CAD build for the part. Positions are in the model's coordinates, mm. A direction names the side the tool comes from. Give positions to 0.01 mm unless a question says otherwise; leave off trailing zeros. Write each loop counter-clockwise with the first axis right and the second up, starting at its lowest first coordinate (ties: lowest second). Pieces come first, ordered by that corner, then holes. Notation, with made-up numbers: M 35.25,-39.75 L 83.25,-39.75 A16 cw 83.25,-13.75 Z; hole C -6.5,9 d1. An arc over 180 degrees is marked long. One line per question, with ' | ' between items. Start each with the question number.
1. Flat gauge pins, fed straight in: pin 1 (0.8 mm diameter, centred on y = -23, z = 1, fed in from +X); pin 2 (17.5 mm diameter, centred on x = -0.5, z = -36.5, fed in from +Y); pin 3 (17.5 mm diameter, centred on y = -7, z = -18, fed in from -X). Where does each tip first touch, or does it go through?
2. Cut at A-A, the plane y = 0. Count the separate pieces of the cut face and the enclosed holes in it, then the cut area to 3 significant figures.
3. Cut at B-B, the plane x = -40. Write the cut outline in (y, z).
4. Cut at D-D, the plane x = -7.5. Write the cut outline in (y, z), then the cut area to 3 significant figures.
5. Which spindle directions (+Z, -Z, +X, -X, +Y, -Y) get a long thin tool onto all of the face, cutting with end or side? Do faces 1 (the face through (0, -17.5, -34)), 2 (the face through (0, 20, -37)), 3 (the face through (20, 0, -37)), 4 (the face through (-20, 0, -37)), 5 (the face through (0, -20, -37)). Say none if no direction does.
6. Cut at C-C, the plane z = -55.5. Write the cut outline in (x, y).
7. Pull direction X, two halves, no side cores. Call faces 6 (the face through (-58, -4, 2.5)), 7 (the face through (60, -1, 5)), 8 (the face through (-35, 0, 1)), 9 (the face through (0, 0, -72.5)): released by +X, released by -X, zero draft, split by the parting line, or undercut.
8. Wall check: L1, parallel to Y at x = 40, z = 1; L2, parallel to X at y = -16, z = -57.5; L3, parallel to X at y = -47.5, z = 3.5. Give the ranges that are in metal, low to high.
```python
from build123d import *

# Parameters (mm, degrees)
F1_W  = 40
F1_H  = 40
F7_W  = 40
F7_H  = 40
F4_W  = 115
F4_H  = 115
F5_W  = 115
F5_H  = 115
F6_W  = 120
F6_H  = 120
F10_W = 120
F10_H = 120
F14_W = 120
F14_H = 120
F12_W = 120
F12_H = 120
F16_T = -2.5
F18_D = 10
F20_D = 10


with BuildPart() as f8:
    # F1 (on offset) → F8 section 0
    with BuildSketch(Plane.XY.offset(-75)):
        Rectangle(F1_W, F1_H)
    # F7 (on Top) → F8 section 1
    with BuildSketch(Plane.XY):
        Rectangle(F7_W, F7_H)
    loft()

    # F4 (on Top) → F9 section 0
    with BuildSketch(Plane.XY):
        Rectangle(F4_W, F4_H)
    # F5 (on offset) → F9 section 1
    with BuildSketch(Plane.XY.offset(2.5)):
        Rectangle(F5_W, F5_H)
    loft()

    # F6 (on offset) → F11 section 0
    with BuildSketch(Plane.XY.offset(5)):
        Rectangle(F6_W, F6_H)
    # F10 (on offset) → F11 section 1
    with BuildSketch(Plane.XY.offset(2.5)):
        Rectangle(F10_W, F10_H)
    loft()

    # F14 (on offset) → F15 section 0
    with BuildSketch(Plane.XY.offset(7.5)):
        Rectangle(F14_W, F14_H)
    # F12 (on face) → F15 section 1
    with BuildSketch(Plane.XY.offset(5)):
        Rectangle(F12_W, F12_H)
    loft()

    # F16
    f16_openings = [f8.faces().sort_by_distance(p)[0] for p in [
        (0, 0, 7.5),
    ]]
    offset(amount=F16_T, openings=f16_openings, kind=Kind.INTERSECTION)

    # F18 (through all)
    with Locations(Plane.XY.offset(2.5)):
        with Locations((-40, 0)):
            Hole(F18_D / 2)

    # F20 (through all)
    with Locations(Plane.XY.offset(2.5)):
        with Locations((40, 0)):
            Hole(F20_D / 2)


solid = f8.part
```
Here are the results:
1) pin 1: x = 57.5 | pin 2: y = 20 | pin 3: x = -20
2) separate pieces: 3 | enclosed holes: 0 | area: 650 mm^2
3) outline: M -60,2.5 L -57.5,2.5 L -57.5,0 L -5,0 L -5,2.5 L -55,2.5 L -55,5 L -57.5,5 L -57.5,7.5 L -60,7.5 Z; M 5,0 L 57.5,0 L 57.5,2.5 L 60,2.5 L 60,7.5 L 57.5,7.5 L 57.5,5 L 55,5 L 55,2.5 L 5,2.5 Z
4) outline: M -60,2.5 L -57.5,2.5 L -57.5,0 L -20,0 L -20,-75 L 20,-75 L 20,0 L 57.5,0 L 57.5,2.5 L 60,2.5 L 60,7.5 L 57.5,7.5 L 57.5,5 L 55,5 L 55,2.5 L 17.5,2.5 L 17.5,-72.5 L -17.5,-72.5 L -17.5,2.5 L -55,2.5 L -55,5 L -57.5,5 L -57.5,7.5 L -60,7.5 Z | area: 700 mm^2
5) face 1: +Z | face 2: -Z, +X, -X, +Y | face 3: -Z, +X, +Y, -Y | face 4: -Z, -X, +Y, -Y | face 5: -Z, +X, -X, -Y
6) outline: M -20,-20 L 20,-20 L 20,20 L -20,20 Z; hole M -17.5,-17.5 L 17.5,-17.5 L 17.5,17.5 L -17.5,17.5 Z
7) face 6: zero draft | face 7: released by +X | face 8: undercut | face 9: undercut
8) L1: -57.5 to -5, 5 to 57.5 | L2: -20 to -17.5, 17.5 to 20 | L3: -60 to -55, 55 to 60
